Autodesk Inventor part; units mm, degrees
ref_plane "YZ Plane" through (0, 0, 0) normal (1, 0, 0) x (0, 1, 0)
ref_plane "XZ Plane" through (0, 0, 0) normal (0, 1, 0) x (-1, 0, 0)
ref_plane "XY Plane" through (0, 0, 0) normal (0, 0, 1) x (1, 0, 0)
sketch "Sketch1" plane through (0, 0, 0) normal (1, 0, 0) x (0, 1, 0)
  line L0 (0, 0) -> (73.993, 0)
  line L1 (0, 130.0359) -> (44.4227, 130.0359)
  line L2 (0, 130.0359) -> (0, 155.2107)
  line L3 (0, 155.2107) -> (44.4227, 155.2107)
  line L4 (44.4227, 155.2107) -> (44.4227, 130.0359)
  line L5 (42.8352, 153.6232) -> (1.5875, 153.6232)
  line L6 (1.5875, 153.6232) -> (1.5875, 131.6234)
  line L7 (1.5875, 131.6234) -> (42.8352, 131.6234)
  line L8 (42.8352, 131.6234) -> (42.8352, 153.6232)
  line L9 (18.2426, 143.1015) -> (18.2426, 119.3292)
  line L10 (14.2738, 131.6234) -> (14.2738, 130.0359)
  line L11 (22.2113, 131.6234) -> (22.2113, 130.0359)
  dimension "d1" = 25.1748
  dimension "d2" = 130.0359
  dimension "d3" = 44.4227
  dimension "d4" = 0
  dimension "d5" = 1.5875
  dimension "d6" = 1.5875
  dimension "d7" = 1.5875
  dimension "d8" = 1.5875
  dimension "d9" = 18.2426
  dimension "d10" = 7.9375
  dimension "d11" = 3.9688
revolve "Revolution1" add sketch "Sketch1" angle 180 about axis through (0, 0, 0) along (0, 1, 0) contours L2 L3 L4 L1 L11 L7 L8 L5 L6 L10
equation "\"d2\" = 0.5 * IBDia - 3 * SpWall"
equation "\"d3\" = Wall + 4 * SpWall + BevDriverDia + d1_1"
equation "\"d5\" = Wall"
equation "\"d6\" = Wall"
equation "\"d7\" = Wall"
equation "\"d8\" = Wall"
equation "\"d9\" = 2 * SpWall + 0.5 * BevDriverDia"
equation "\"d10\" = AxelDia + Space"
equation "\"d11\" = 0.5 * Space + 0.5 * AxelDia"
equation "\"IDia\" = 266.7"
equation "\"Wall\" = 1.5875"
equation "\"Space\" = 1.5875"
equation "\"SpWall\" = 3.175"
equation "\"AxelDia\" = 6.35"
properties part number "OuterShell"
Geometry: final body of the model. Coordinates: model frame, mm. A direction names the side the tool comes from. Coordinates: 2 decimals unless noted, no trailing zeros. Order: outer loops, then holes, each group sorted by start corner. A loop starts at its lowest first (then second) coordinate and runs counter-clockwise, first axis right, second up.
Item 1: Section query B-B (y = 6). Output: boundary loops of the cut face in (x, z).
Answer:
outline: (0, -155.21) arc R155.21 ccw to (0, 155.21) - (0, 153.62) arc R153.62 cw to (0, -153.62) - close; (0, -131.62) arc R131.62 ccw to (0, 131.62) - (0, 130.04) arc R130.04 cw to (0, -130.04) - close
Item 2: Section query D-D (x = 32). Output: boundary loops of the cut face in (y, z).
Answer:
outline: (0, -151.88) - (44.42, -151.88) - (44.42, -126.04) - (22.21, -126.04) - (22.21, -127.67) - (42.84, -127.67) - (42.84, -150.25) - (1.59, -150.25) - (1.59, -127.67) - (14.27, -127.67) - (14.27, -126.04) - (0, -126.04) - close; (0, 126.04) - (14.27, 126.04) - (14.27, 127.67) - (1.59, 127.67) - (1.59, 150.25) - (42.84, 150.25) - (42.84, 127.67) - (22.21, 127.67) - (22.21, 126.04) - (44.42, 126.04) - (44.42, 151.88) - (0, 151.88) - close
Item 3: Access query for faces 1 (the face through (131.59, 32.67, 2.89)), 2 (the face through (130, 0, 11)), 3 (the face through (129, 22.211, 19)). Directions: +Z, -Z, +X, -X, +Y, -Y. A direction counts if a zero-diameter tool reaches every point of the face in a straight line with its end or side. Return the directions, or none.
Answer:
face 1: none
face 2: +Z, -Z, +X, -X, -Y
face 3: -X
Item 4: Draft query along X for faces 4 (the face through (155.173, 22.522, 3.413)), 5 (the face through (130, 7, 3)), 6 (the face through (134, 42.835, 11)). Return one class per face: released by +X, released by -X, zero draft, split by the parting line, or undercut.
Answer:
face 4: released by +X
face 5: released by -X
face 6: undercut
Item 5: Section query A-A (x = 82). Output: boundary loops of the cut face in (y, z).
Answer:
outline: (0, -131.78) - (44.42, -131.78) - (44.42, -100.92) - (22.21, -100.92) - (22.21, -102.96) - (42.84, -102.96) - (42.84, -129.91) - (1.59, -129.91) - (1.59, -102.96) - (14.27, -102.96) - (14.27, -100.92) - (0, -100.92) - close; (0, 100.92) - (14.27, 100.92) - (14.27, 102.96) - (1.59, 102.96) - (1.59, 129.91) - (42.84, 129.91) - (42.84, 102.96) - (22.21, 102.96) - (22.21, 100.92) - (44.42, 100.92) - (44.42, 131.78) - (0, 131.78) - close
Item 6: Material intervals for line 1 along Y through (x, z) = (63, -131); line 2 along X through (y, z) = (7, 2); line 3 along Z through (x, y) = (89.5, 38.5), sorted ascending.
Answer:
line 1: y = 0 to 1.59, 42.84 to 44.42
line 2: x = 130.02 to 131.61, 153.61 to 155.2
line 3: z = -126.81 to -124.86, -96.51 to -94.33, 94.33 to 96.51, 124.86 to 126.81
Item 7: Section query C-C (z = 0). Output: boundary loops of the cut face in (x, y), then the cut area to 3 significant figures.
Answer:
outline: (130.04, 0) - (155.21, 0) - (155.21, 44.42) - (130.04, 44.42) - (130.04, 22.21) - (131.62, 22.21) - (131.62, 42.84) - (153.62, 42.84) - (153.62, 1.59) - (131.62, 1.59) - (131.62, 14.27) - (130.04, 14.27) - close
area: 198 mm2
Item 8: Contact query for flat-ended pins moving along their axis: P1, Ø5, axis at x = 129.5, y = 9, coming from the +Z side; P2, Ø6, axis at y = 8, z = 42.5, coming from the +X side; P3, Ø2, axis at y = 12.5, z = 120, coming from the +X side. Output: stop coordinate, or through.
Answer:
P1: stops at z = 89.23
P2: stops at x = 150.1
P3: stops at x = 99.65
